```python
from build123d import *

# Parameters (mm, degrees)
SKETCH3_R          = 4
CUT_EXTRUDE1_DEPTH = 22
SKETCH4_R          = 4.5
CUT_EXTRUDE2_DEPTH = 32


with BuildPart() as part:
    # Sketch2 → Revolve1 (revolve)
    with BuildSketch(Plane.XY, mode=Mode.PRIVATE) as revolve1_sk:
        Polygon((-14.2, 18.5), (-4, 18.5), (-4, 37.173414273), (-5.326585727, 38.5), (-14.2, 35.5), align=None)
    revolve(revolve1_sk.sketch.rotate(Axis((0, 15.2, 0), (0, 1, 0)), 270), axis=Axis((0, 15.2, 0), (0, 1, 0)))

    # Sketch3 → Cut-Extrude1 (cut)
    with BuildSketch(Plane(origin=(0, 0, 0), x_dir=(0, 0, -1), z_dir=(1, 0, 0))):
        with Locations((0, 27.7)):
            Circle(SKETCH3_R)
    extrude(amount=-CUT_EXTRUDE1_DEPTH, mode=Mode.SUBTRACT)

    # Sketch4 → Cut-Extrude2 (cut)
    with BuildSketch(Plane.XZ.offset(-18.5)):
        with Locations(Location((0, 0, 0), (0, 0, 270))):
            Circle(SKETCH4_R)
    extrude(amount=-CUT_EXTRUDE2_DEPTH, mode=Mode.SUBTRACT)


solid = part.part
```
For this review, take the finished solid that the model builds, in its own axes (mm). A direction names the side the tool comes from. Give positions to 0.01 mm unless a question says otherwise; leave off trailing zeros. Order: outer loops, then holes, each group sorted by start corner. A loop starts at its lowest first (then second) coordinate and runs counter-clockwise, first axis right, second up.
1) Take a section at A-A (z = 0). Give the boundary of the cut face in (x, y), then the cut area to 3 significant figures.
2) Take a section at D-D (z = -3.5). State how many separate pieces and enclosed holes the cut face has, then the cut area to 3 significant figures.
3) Take a section at C-C (y = 27.7). Give the boundary of the cut face in (x, z).
4) Take a section at B-B (y = 36.25). Give the boundary of the cut face in (x, z).
5) The part is to be moulded in two halves that separate along X. For faces 1 (the face through (-3.4, 18.5, 3.4)), 2 (the face through (5.742, 38.312, 1.275)), 3 (the face through (4.46, 27.95, 0.59)), say which applies: released by +X, released by -X, zero draft, split by the parting line, or undercut.
6) Wall thickness on line 1 (X direction, y = 32.75, z = 0); line 2 (Y direction, x = -7.75, z = 0); line 3 (Z direction, x = -3, y = 32.75): over which ranges is each line inside the solid? List them lowest first.
7) For faces 4 (the face through (-8.046, 31.073, -2.15)), 5 (the face through (12.6, 26.88, -6.55)), list the 3-axis set-ups (+Z, -Z, +X, -X, +Y, -Y) from which the entire face can be reached by the end or side of a thin tool; tool diameter is ignored.
8) Insertion check: pin 1 (1.5 mm diameter, centred on x = -11, z = -5.5, fed in from +Y); pin 2 (1 mm diameter, centred on x = -11, y = 22.5, fed in from +Z); pin 3 (3 mm diameter, centred on x = 5.5, y = 34, fed in from +Z) (3 decimals). Each pin has a flat end and moves straight along its axis. Give the tip position at first contact, or say it passes through.
Derived:
1. outline: (-14.2, 18.5) - (-4.5, 18.5) - (-4.5, 23.7) - (-14.2, 23.7) - close; (-14.2, 31.7) - (-4.5, 31.7) - (-4.5, 37.67) - (-5.33, 38.5) - (-14.2, 35.5) - close; (4.5, 18.5) - (14.2, 18.5) - (14.2, 35.5) - (5.33, 38.5) - (4.5, 37.67) - close
1. area: 283 mm2
2. separate pieces: 3
2. enclosed holes: 0
2. area: 366 mm2
3. outline: (-13.62, -4) arc R14.2 ccw (long way) to (-13.62, 4) - (-2.06, 4) arc R4.5 cw (long way) to (-2.06, -4) - close
4. outline: circle Ø23.96 at (0, 0); hole circle Ø9 at (0, 0)
5. face 1: zero draft
5. face 2: split by the parting line
5. face 3: undercut
6. line 1: x = -14.2 to -4.5, 4.5 to 14.2
6. line 2: y = 18.5 to 23.7, 31.7 to 37.68
6. line 3: z = -13.88 to -3.35, 3.35 to 13.88
7. face 4: -X
7. face 5: +Y, -Y
8. pin 1: stops at y = 36.4
8. pin 2: stops at z = 9.56
8. pin 3: stops at z = 13.625
